For this review, take the finished solid that the model builds, in its own axes (mm). A direction names the side the tool comes from. Coordinates: 2 decimals unless noted, no trailing zeros. Write each loop counter-clockwise with the first axis right and the second up, starting at its lowest first coordinate (ties: lowest second). Pieces come first, ordered by that corner, then holes.
```python
from build123d import *

# Parameters (mm, degrees)
SKETCH_W     = 45
SKETCH_H     = 40
PAD_DEPTH    = 5
SKETCH001_W  = 41.2
SKETCH001_H  = 36.2
POCKET_DEPTH = 4
FILLET_R     = 1


with BuildPart() as part:
    # Sketch → Pad (new body)
    with BuildSketch(Plane.XY):
        Rectangle(SKETCH_W, SKETCH_H)
    extrude(amount=PAD_DEPTH)

    # Sketch001 (on Face6 of Pad) → Pocket (cut)
    with BuildSketch(Plane.XY.offset(5)):
        Rectangle(SKETCH001_W, SKETCH001_H)
    extrude(amount=-POCKET_DEPTH, mode=Mode.SUBTRACT)

    # Fillet
    fillet_edges = [part.edges().sort_by_distance(p)[0] for p in [
        (0, 20, 0),
        (22.5, 0, 0),
        (0, -20, 0),
        (-22.5, 0, 0),
    ]]
    fillet(fillet_edges, radius=FILLET_R)


solid = part.part
```
Q1. Tool access review of faces 1 (the flat face through (0, 0, 1)), 2 (the cylindrical face through (0.315, -19.715, 0.301)): name each direction out of +Z, -Z, +X, -X, +Y, -Y from which nothing blocks a thin tool from reaching the whole face with its end or side.
Ans:
face 1: +Z
face 2: -Z, +X, -X, -Y
Q2. For probe 1 along X at (y, z) = (-7.5, 1.2); probe 2 along Y at (x, z) = (-2, 4.4); probe 3 along Z at (x, y) = (-14, -12.5), list the stretches that pass through material, from the lowest coordinate up.
Ans:
probe 1: x = -22.5 to -20.6, 20.6 to 22.5
probe 2: y = -20 to -18.1, 18.1 to 20
probe 3: z = 0 to 1
Q3. Add section C-C (x = -15). State the section outline as (y, z) points, then the cut area to 3 significant figures.
Ans:
outline: (-20, 1) arc R1 ccw to (-19, 0) - (19, 0) arc R1 ccw to (20, 1) - (20, 5) - (18.1, 5) - (18.1, 1) - (-18.1, 1) - (-18.1, 5) - (-20, 5) - close
area: 54.8 mm2
Q4. Add section A-A (z = 3.2). State the section outline as (x, y) points, then the cut area to 3 significant figures.
Ans:
outline: (-22.5, -20) - (22.5, -20) - (22.5, 20) - (-22.5, 20) - close; hole (-20.6, -18.1) - (20.6, -18.1) - (20.6, 18.1) - (-20.6, 18.1) - close
area: 309 mm2
Q5. Clearance check with a flat-ended pin moving along its axis: pin 1 Ø11 at (x, y) = (-7, 6) entering from +Z. State where the tip first meets the part, or that it passes through.
Ans:
pin 1: stops at z = 1
Q6. Draft analysis for pull direction X (two halves, no side actions). For faces 3 (the flat face through (-22.5, 0, 3)), 4 (the flat face through (0, 0, 0)), 5 (the flat face through (0, -18.1, 3)), state which applies: +X half, -X half, draft (parallel to the pull), parting line (faces both ways), or undercut.
Ans:
face 3: -X half
face 4: draft
face 5: undercut
Q7. Add section B-B (y = 7). State the section outline as (x, z) points.
Ans:
outline: (-22.5, 1) arc R1 ccw to (-21.5, 0) - (21.5, 0) arc R1 ccw to (22.5, 1) - (22.5, 5) - (20.6, 5) - (20.6, 1) - (-20.6, 1) - (-20.6, 5) - (-22.5, 5) - close
